```python
from build123d import *

# Parameters (mm, degrees)
F1_DEPTH = 32
F2_R     = 2.54
F3_DEPTH = 25.4
F4_R     = 2.54
F5_DEPTH = 25.4


with BuildPart() as f1:
    # F0 (on Front) → F1 (new body)
    with BuildSketch(Plane.XZ):
        Polygon((-15, 15.75), (-16, 15.75), (-16, -16.25), (16, -16.25), (16, -15.25), (-15, -15.25), align=None)
    extrude(amount=F1_DEPTH)

    # F2 (on face) → F3 (cut)
    with BuildSketch(Plane(origin=(-16, 0, 0), x_dir=(0, -1, 0), z_dir=(-1, 0, 0))):
        with Locations((16, -0.25)):
            Circle(F2_R)
    extrude(amount=-F3_DEPTH, mode=Mode.SUBTRACT)

    # F4 (on face) → F5 (cut)
    with BuildSketch(Plane(origin=(0, 0, -16.25), x_dir=(1, 0, 0), z_dir=(0, 0, -1))):
        with Locations((0, 16)):
            Circle(F4_R)
    extrude(amount=-F5_DEPTH, mode=Mode.SUBTRACT)


solid = f1.part
```
Work out the finished part from the listing and answer in its coordinate system (mm). A direction names the side the tool comes from. Coordinates: 2 decimals unless noted, no trailing zeros. Order: outer loops, then holes, each group sorted by start corner. A loop starts at its lowest first (then second) coordinate and runs counter-clockwise, first axis right, second up. Notation, with made-up numbers: (-29.5, 56) - (14.5, 56) arc R12 cw to (14.5, 68) - close; hole circle Ø4 at (76, 15). An arc over 180 degrees is marked (long way). Answer as a JSON object with one key per item and string values.
1. Find section C-C on z = -0.25. Determine the outline of the cut face in (x, y), plus the area to 3 significant figures.
Output values:
{"outline": "(-16, -32) - (-15, -32) - (-15, -18.54) - (-16, -18.54) - close; (-16, -13.46) - (-15, -13.46) - (-15, 0) - (-16, 0) - close", "area": "26.9 mm²"}
2. Find section D-D on y = -11.5. Determine the outline of the cut face in (x, z), plus the area to 3 significant figures.
Output values:
{"outline": "(-16, -16.25) - (16, -16.25) - (16, -15.25) - (-15, -15.25) - (-15, 15.75) - (-16, 15.75) - close", "area": "63.0 mm²"}
3. Each of these flat-tipped pins is pushed along its axis until it touches: P1, Ø9.5, axis at y = -23.5, z = 3.5, coming from the +X side; P2, Ø8, axis at x = 0, y = -16, coming from the -Z side. Where does it stop, or does it pass through?
Output values:
{"P1": "stops at x = -15", "P2": "stops at z = -16.25"}
4. A tool of negligible diameter and unlimited length cuts with its end or side. For faces 4 (the face through (-15, -16, 3)), 5 (the face through (-15.5, -32, -7.3)), from which of +Z, -Z, +X, -X, +Y, -Y can it reach the whole face along a straight path? Write none if from no direction.
Output values:
{"face 4": "+Z, +X, +Y, -Y", "face 5": "+Z, -Z, +X, -X, -Y"}
5. Find section B-B on x = 0. Determine the outline of the cut face in (y, z), plus the area to 3 significant figures.
Output values:
{"outline": "(-32, -16.25) - (-18.54, -16.25) - (-18.54, -15.25) - (-32, -15.25) - close; (-13.46, -16.25) - (0, -16.25) - (0, -15.25) - (-13.46, -15.25) - close", "area": "26.9 mm²"}
6. The mould has two halves that part along Z. Classify faces 1 (the face through (-15.507, -18.346, -1.223)), 2 (the face through (-0.55, -13.52, -15.76)), 3 (the face through (0, -12, -16.25)): +Z half, -Z half, draft (parallel to the pull), parting line (faces both ways), or undercut.
Output values:
{"face 1": "undercut", "face 2": "draft", "face 3": "-Z half"}
7. Find section A-A on y = -16. Determine the outline of the cut face in (x, z), plus the area to 3 significant figures.
Output values:
{"outline": "(-16, -16.25) - (-2.54, -16.25) - (-2.54, -15.25) - (-15, -15.25) - (-15, -2.79) - (-16, -2.79) - close; (-16, 2.29) - (-15, 2.29) - (-15, 15.75) - (-16, 15.75) - close; (2.54, -16.25) - (16, -16.25) - (16, -15.25) - (2.54, -15.25) - close", "area": "52.8 mm²"}
8. Consider line 1 (Z direction, x = -15.5, y = -16); line 2 (Z direction, x = -11.5, y = -16.5); line 3 (X direction, y = -27.5, z = 14). Determine where each line is inside the solid, lowest interval first.
Output values:
{"line 1": "z = -16.25 to -2.79, 2.29 to 15.75", "line 2": "z = -16.25 to -15.25", "line 3": "x = -16 to -15"}
